Input: part model. Units: mm. Frame: model coordinates. A direction names the side the tool comes from. Round coordinates to 2 decimals unless told otherwise and drop trailing zeros. Order: outer loops, then holes, each group sorted by start corner. A loop starts at its lowest first (then second) coordinate and runs counter-clockwise, first axis right, second up. Notation, with made-up numbers: (15.5, 87) - (69.5, 87) arc R16 cw to (69.5, 97) - close; hole circle Ø4 at (37, -35). An arc over 180 degrees is marked (long way). One line per item, written item: value. Start each with the question number.
from build123d import *

# Parameters (mm, degrees)
F0_W     = 254
F0_H     = 1219.2
F1_DEPTH = 914.4
F3_DEPTH = 254.001
F5_DEPTH = 254.001
F6_F1_R  = 12.7
F6_F2_R  = 12.7


with BuildPart() as f1:
    # F0 (on Front) → F1 (new body)
    with BuildSketch(Plane.XZ):
        with Locations((-127, 609.6)):
            Rectangle(F0_W, F0_H)
    extrude(amount=F1_DEPTH)

    # F2 (on Right) → F3 (cut, through all)
    with BuildSketch(Plane.YZ):
        Polygon((-462.4002873898, 1231.0378551483), (0, 0), (0, 1231.0378551483), align=None)
    extrude(amount=-F3_DEPTH, mode=Mode.SUBTRACT)

    # F4 (on Right) → F5 (cut, through all)
    with BuildSketch(Plane.YZ):
        Polygon((-437.4758601189, 0), (-32.0333614945, 0), (-481.8673729897, 1177.9962778091), align=None)
    extrude(amount=-F5_DEPTH, mode=Mode.SUBTRACT)

    # F6: fillet of radius 12.7 on 8 edges, made by hand

    # F6_f1
    f6_f1_edges = [f1.edges().sort_by_distance(p)[0] for p in [
        (-127, -481.8673729897, 1177.9962778091),
    ]]
    fillet(f6_f1_edges, radius=F6_F1_R)

    # F6_f2
    f6_f2_edges = [f1.edges().sort_by_distance(p)[0] for p in [
        (-127, -914.4, 0),
        (0, -914.4, 609.6),
        (-127, -914.4, 1219.2),
        (-254, -914.4, 609.6),
        (0, -458.2226343973, 550.5471946336),
        (-127, -437.4758601189, 0),
        (-254, -458.2226343973, 550.5471946336),
        (-254, -468.8167042617, 1114.0163928436),
        (0, -468.8167042617, 1114.0163928436),
    ]]
    fillet(f6_f2_edges, radius=F6_F2_R)


solid = f1.part
1. Section A-A (x = -174.5). Return the cut outline in (y, z).
2. Pin query (flat end, axial travel): pin 1 (10 mm diameter, centred on x = -194, z = 1048, fed in from +Y); pin 2 (4 mm diameter, centred on x = -210.5, z = 404.5, fed in from +Y); pin 3 (5 mm diameter, centred on x = -90.5, z = 632.5, fed in from +Y). Return the tip coordinate at first contact, or that it passes through.
3. Line query: line 1 (Y direction, x = -80, z = 95.5); line 2 (Y direction, x = -100.5, z = 73.5). Output: solid intervals per line, ascending. Write a range as from..to.
4. Pull-direction query (Z, two-part tool) for faces 4 (the face through (-129, -677, 1219.2)), 5 (the face through (0, -645, 601)), 6 (the face through (-129, -16, 0)), 7 (the face through (-128.6, -469.061, 1113.964)); classes: released by +Z, released by -Z, zero draft, split by the parting line, or undercut.
5. Set-up query: faces 1 (the face through (-250.38, -462.34, 558.35)), 2 (the face through (-125.4, -458.758, 564.752)), 3 (the face through (-3.82, -461.56, 542.95)). Return all of +Z, -Z, +X, -X, +Y, -Y with unobstructed straight access to the full face (end or side cutting, diameter ignored); none if empty.
Solved:
1. outline: (-914.4, 12.7) arc R12.7 ccw to (-901.7, 0) - (-450.66, 0) arc R12.7 ccw to (-437.97, 13.18) - (-478.97, 1101.09) arc R12.7 cw to (-454.41, 1106.1) - (-32.03, 0) - (0, 0) - (-457.95, 1219.2) - (-901.7, 1219.2) arc R12.7 ccw to (-914.4, 1206.5) - close
2. pin 1: stops at y = -391.77
2. pin 2: stops at y = -151.19
2. pin 3: stops at y = -236.64
3. line 1: y = -914.4..-441.07, -68.5..-35.87
3. line 2: y = -914.4..-440.25, -60.1..-27.61
4. face 4: released by +Z
4. face 5: zero draft
4. face 6: released by -Z
4. face 7: undercut
5. face 1: -X
5. face 2: +X, -X
5. face 3: +X
